Work out the finished part from the listing and answer in its coordinate system (mm). A direction names the side the tool comes from. Give positions to 0.01 mm unless a question says otherwise; leave off trailing zeros. Loops run counter-clockwise (first coordinate to the right, second up) from the corner with the lowest first, then second, coordinate; pieces in that order, holes last. Notation, with made-up numbers: (47.25, 25.5) - (71.25, 25.5) arc R5 cw to (71.25, 30.5) - close; hole circle Ø5 at (-12.75, 55). An arc over 180 degrees is marked (long way). One line per item, written item: value.
from build123d import *

# Parameters (mm, degrees)
SKETCH1_W                                    = 25.5
SKETCH1_H                                    = 36
BOSS_EXTRUDE1_DEPTH                          = 4
CUT_EXTRUDE1_REACH                           = 40.4
SKETCH2_W                                    = 12
SKETCH2_H                                    = 1.5
CSK_FOR_M5_COUNTERSUNK_FLAT_HEAD_SCR_2_COUNT = 2
CSK_FOR_M5_COUNTERSUNK_FLAT_HEAD_SCR_2_PITCH = 20
M3_CLEARANCE_HOLE1_D                         = 3.1
HOLE1_D                                      = 4.2
FILLET1_R                                    = 1


with BuildPart() as part:
    # Sketch1 → Boss-Extrude1 (new body)
    with BuildSketch(Plane.XY):
        Rectangle(SKETCH1_W, SKETCH1_H)
    extrude(amount=BOSS_EXTRUDE1_DEPTH)

    # Sketch2 → Cut-Extrude1 (cut, up to next)
    with BuildSketch(Plane(origin=(0, 18, 0), x_dir=(1, 0, 0), z_dir=(0, 1, 0)), mode=Mode.PRIVATE) as cut_extrude1_sk1:
        with Locations((-6.75, -0.75)):
            Rectangle(SKETCH2_W, SKETCH2_H)
    cut_extrude1_tool1 = extrude(cut_extrude1_sk1.sketch, amount=-CUT_EXTRUDE1_REACH, mode=Mode.PRIVATE) & part.part
    add(cut_extrude1_tool1.solids().sort_by_distance((-6.75, 18, 0.75))[0], mode=Mode.SUBTRACT)

    # Sketch5 → CSK for M5 Countersunk Flat Head Screw1 (revolve, cut)
    with BuildSketch(Plane(origin=(4.75, 10, 0), x_dir=(0, 1, 0), z_dir=(1, 0, 0))):
        Polygon((0, 0), (0, 4), (2.775, 4), (2.75, 3.975), (2.75, 2.45), (5.2, 0), align=None)
    csk_for_m5_countersunk_flat_head_screw1 = revolve(axis=Axis((4.75, 10, -6.35), (0, 0, 1)), mode=Mode.SUBTRACT)

    # CSK for M5 Countersunk Flat Head Scr 2: CSK for M5 Countersunk Flat Head Screw1 ×2
    with Locations(*[(0, -i * CSK_FOR_M5_COUNTERSUNK_FLAT_HEAD_SCR_2_PITCH, 0) for i in range(1, CSK_FOR_M5_COUNTERSUNK_FLAT_HEAD_SCR_2_COUNT)]):
        add(csk_for_m5_countersunk_flat_head_screw1, mode=Mode.SUBTRACT)

    # M3 Clearance Hole1 (through all)
    with Locations(Plane(origin=(0, 0, 1.5), x_dir=(-1, 0, 0), z_dir=(0, 0, -1))):
        with Locations((9.75, -15.35)):
            Hole(M3_CLEARANCE_HOLE1_D / 2)

    # Hole1 (through all)
    with Locations(Plane(origin=(0, 0, 1.5), x_dir=(-1, 0, 0), z_dir=(0, 0, -1))):
        with Locations((9.75, -2.3)):
            Hole(HOLE1_D / 2)

    # Fillet1
    fillet1_edges = [part.edges().sort_by_distance(p)[0] for p in [
        (-12.75, 18, 2.75),
        (12.75, 18, 2),
        (12.75, -18, 2),
        (-12.75, -18, 2.75),
    ]]
    fillet(fillet1_edges, radius=FILLET1_R)


solid = part.part
1. Flat-ended cylindrical pins translate along their axes: pin 1 Ø7 at (x, y) = (4.75, 10) entering from +Z; pin 2 Ø1.2 at (y, z) = (-3.5, 0.5) entering from -X; pin 3 Ø2.5 at (x, y) = (-9.75, -2.3) entering from -Z; pin 4 Ø3.5 at (x, y) = (-9.75, -15.35) entering from -Z. Find the tip coordinate at first contact, or state that the pin passes through.
Output:
pin 1: stops at z = 4
pin 2: stops at x = -0.75
pin 3: passes through
pin 4: stops at z = 1.5
2. Section D-D (z = 3.1) is taken. Write down the section's boundary in (x, y).
Output:
outline: (-12.75, -17) arc R1 ccw to (-11.75, -18) - (11.75, -18) arc R1 ccw to (12.75, -17) - (12.75, 17) arc R1 ccw to (11.75, 18) - (-11.75, 18) arc R1 ccw to (-12.75, 17) - close; hole circle Ø4.2 at (-9.75, -2.3); hole circle Ø3.1 at (-9.75, -15.35); hole circle Ø5.5 at (4.75, -10); hole circle Ø5.5 at (4.75, 10)
3. For faces 1 (the flat face through (-0.75, 0, 1)), 2 (the flat face through (12.75, 0, 2)), determine the directions among +Z, -Z, +X, -X, +Y, -Y from which every point of the face is accessible in a straight line to the end or side of a thin tool.
Output:
face 1: -Z, -X, +Y, -Y
face 2: +Z, -Z, +X, +Y, -Y
4. Section A-A (x = 4.75) is taken. Write down the section's boundary in (y, z) (3 decimals), and give its area (3 significant figures).
Output:
outline: (-18, 0) - (-15.2, 0) - (-12.75, 2.45) - (-12.75, 3.975) - (-12.775, 4) - (-18, 4) - close; (-7.25, 2.45) - (-4.8, 0) - (4.8, 0) - (7.25, 2.45) - (7.25, 3.975) - (7.225, 4) - (-7.225, 4) - (-7.25, 3.975) - close; (12.75, 2.45) - (15.2, 0) - (18, 0) - (18, 4) - (12.775, 4) - (12.75, 3.975) - close
area: 88.0 mm²
5. Find the intervals of material crossed by line 1 along Y through (x, z) = (-9.75, 2.3); line 2 along Y through (x, z) = (4.75, 3.3); line 3 along X through (y, z) = (10, 3.3), in increasing order.
Output:
line 1: y = -18 to -16.9, -13.8 to -4.4, -0.2 to 18
line 2: y = -18 to -12.75, -7.25 to 7.25, 12.75 to 18
line 3: x = -12.75 to 2, 7.5 to 12.75
6. Section C-C (z = 1) is taken. Write down the section's boundary in (x, y), and give its area (3 significant figures).
Output:
outline: (-0.75, -18) - (11.75, -18) arc R1 ccw to (12.75, -17) - (12.75, 17) arc R1 ccw to (11.75, 18) - (-0.75, 18) - close; hole circle Ø8.4 at (4.75, -10); hole circle Ø8.4 at (4.75, 10)
area: 375 mm²
7. Section B-B (y = -2.3) is taken. Write down the section's boundary in (x, z), and give its area (3 significant figures).
Output:
outline: (-12.75, 1.5) - (-11.85, 1.5) - (-11.85, 4) - (-12.75, 4) - close; (-7.65, 1.5) - (-0.75, 1.5) - (-0.75, 0) - (12.75, 0) - (12.75, 4) - (-7.65, 4) - close
area: 73.5 mm²
